from build123d import *

# Parameters (mm, degrees)
SKETCH1_W           = 42
SKETCH1_H           = 38
BOSS_EXTRUDE1_DEPTH = 20
SKETCH3_R           = 1.995914713
BOSS_EXTRUDE2_DEPTH = 2
SKETCH4_W           = 20
SKETCH4_H           = 4.118584071
BOSS_EXTRUDE3_DEPTH = 7.5


with BuildPart() as part:
    # Sketch1 → Boss-Extrude1 (new body)
    with BuildSketch(Plane.XY):
        Rectangle(SKETCH1_W, SKETCH1_H)
    extrude(amount=BOSS_EXTRUDE1_DEPTH)

    # Sketch3 → Boss-Extrude2 (add)
    with BuildSketch(Plane(origin=(0, 19, 0), x_dir=(1, 0, 0), z_dir=(0, 1, 0))):
        with Locations(Location((-10.84, -10, 0), (0, 0, 270))):
            Circle(SKETCH3_R)
    extrude(amount=BOSS_EXTRUDE2_DEPTH)

    # Sketch4 → Boss-Extrude3 (add)
    with BuildSketch(Plane.ZY.offset(21)):
        with Locations((10, 16.940707964)):
            Rectangle(SKETCH4_W, SKETCH4_H)
    boss_extrude3 = extrude(amount=BOSS_EXTRUDE3_DEPTH)

    # Mirror2: Boss-Extrude3 across plane
    add(boss_extrude3.mirror(Plane(origin=(0, 0, 0), x_dir=(0, 0, 1), z_dir=(1, 0, 0))))


solid = part.part
Geometry check sheet. Reference: the model listing, model coordinates, mm. A direction names the side the tool comes from. Give positions to 0.01 mm unless a question says otherwise; leave off trailing zeros. Write each loop counter-clockwise with the first axis right and the second up, starting at its lowest first coordinate (ties: lowest second). Pieces come first, ordered by that corner, then holes. Notation, with made-up numbers: M 48,85.5 L 68,85.5 A21 ccw 68,123.5 Z; hole C -20.75,64 d9. An arc over 180 degrees is marked long. Answer as CSV lines item,"result". Start each with the question number.
Q1. Section check A-A, the plane z = 18. Record the cut outline in (x, y).
Q2. Go/stop test with flat-tipped pins: pin 1 (1 mm diameter, centred on y = 1, z = 12.5, fed in from +X); pin 2 (8 mm diameter, centred on x = 5.5, z = 7.5, fed in from +Y); pin 3 (4 mm diameter, centred on y = -1.5, z = 13.5, fed in from -X). Record where each tip stops, or that it passes through.
Q3. Tool access check on faces 4 (the face through (25, 14.881, 10)), 5 (the face through (-21, -2, 10)), 6 (the face through (-28.5, 17, 10)). Record the directions out of +Z, -Z, +X, -X, +Y, -Y that give a thin tool (end or side, any length) a straight path to the whole face; none if there is none.
Q4. Section check B-B, the plane x = -10.84. Record the cut outline in (y, z), then the cut area to 3 significant figures.
Q5. Section check C-C, the plane y = -5. Record the cut outline in (x, z).
Q6. Section check D-D, the plane z = 10. Record the cut outline in (x, y).
Q7. Release check for a two-part mould opening along X. For faces 1 (the face through (0, -19, 10)), 2 (the face through (-12.61, 19.99, 10.92)), 3 (the face through (28.5, 17, 10)) record: pulls with the +X half, pulls with the -X half, needs draft (parallel to the pull), parting line crosses it, or undercut.
Q8. Material ranges on L1, parallel to X at y = -1, z = 13.75; L2, parallel to Y at x = -11, z = 12.5; L3, parallel to Y at x = -25, z = 3, recorded low to high.
Geometry says:
1,outline,"M -28.5,14.88 L -21,14.88 L -21,-19 L 21,-19 L 21,14.88 L 28.5,14.88 L 28.5,19 L -28.5,19 Z"
2,pin 1,"x = 21"
2,pin 2,"y = 19"
2,pin 3,"x = -21"
3,face 4,"+Z, -Z, +X, -Y"
3,face 5,"+Z, -Z, -X, -Y"
3,face 6,"+Z, -Z, -X, +Y, -Y"
4,outline,"M -19,0 L 19,0 L 19,8 L 21,8 L 21,12 L 19,12 L 19,20 L -19,20 Z"
4,area,"768 mm^2"
5,outline,"M -21,0 L 21,0 L 21,20 L -21,20 Z"
6,outline,"M -28.5,14.88 L -21,14.88 L -21,-19 L 21,-19 L 21,14.88 L 28.5,14.88 L 28.5,19 L -8.84,19 L -8.84,21 L -12.84,21 L -12.84,19 L -28.5,19 Z"
7,face 1,"needs draft"
7,face 2,"parting line crosses it"
7,face 3,"pulls with the +X half"
8,L1,"-21 to 21"
8,L2,"-19 to 19"
8,L3,"14.88 to 19"
